Verification items for the finished model (mm, model axes). Give positions to 0.01 mm unless a question says otherwise; leave off trailing zeros. Write each loop counter-clockwise with the first axis right and the second up, starting at its lowest first coordinate (ties: lowest second). Pieces come first, ordered by that corner, then holes. Notation, with made-up numbers: M 12,59 L 21,59 A13 cw 21,83 Z; hole C -31,-34.75 d10. An arc over 180 degrees is marked long. Write item = value, one per line.
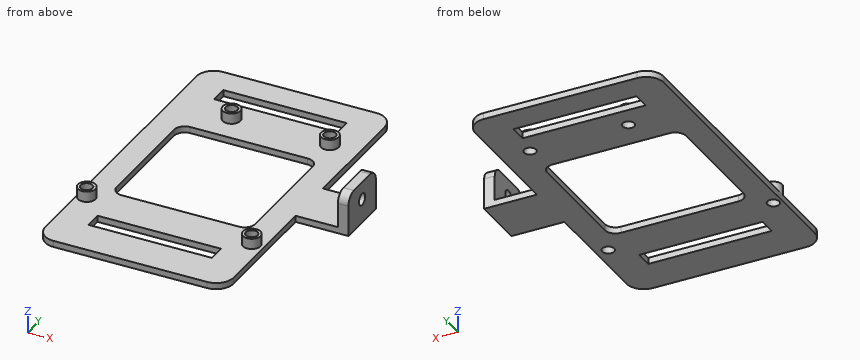
from build123d import *

# Parameters (mm, degrees)
SKETCH_W        = 53.5
SKETCH_H        = 92.8
PAD_DEPTH       = 1.8
SKETCH001_R     = 2.5
PAD001_DEPTH    = 3
SKETCH002_R     = 1.7
POCKET_DEPTH    = 5
SKETCH003_W     = 15
SKETCH003_H     = 1.8
PAD002_DEPTH    = 15
SKETCH004_W     = 39.320262
SKETCH004_H     = 37.514924
POCKET001_DEPTH = 5
FILLET_R        = 5
FILLET001_R     = 5
SKETCH005_W     = 35
SKETCH005_H     = 5
POCKET002_DEPTH = 5
SKETCH006_W     = 3
SKETCH006_H     = 15
PAD003_DEPTH    = 10
SKETCH007_R     = 1.7
POCKET003_DEPTH = 5
FILLET002_R     = 5
FILLET003_R     = 5
FILLET004_R     = 3
FILLET005_R     = 3
FILLET006_R     = 3
FILLET007_R     = 3
FILLET008_R     = 3
FILLET009_R     = 3


with BuildPart() as part:
    # Sketch → Pad (new body)
    with BuildSketch(Plane.XY):
        with Locations((0.1, 0)):
            Rectangle(SKETCH_W, SKETCH_H)
    extrude(amount=PAD_DEPTH)

    # Sketch001 (on Face6 of Pad) → Pad001 (join)
    with BuildSketch(Plane.XY.offset(1.8)):
        with Locations((-9.25, 27.14)):
            Circle(SKETCH001_R)
        with Locations((18.65, 27.14)):
            Circle(SKETCH001_R)
        with Locations((-24.132207, -23.46)):
            Circle(SKETCH001_R)
        with Locations((23.35, -24.76)):
            Circle(SKETCH001_R)
    extrude(amount=PAD001_DEPTH)

    # Sketch002 (on Face12 of Pad001) → Pocket (cut)
    with BuildSketch(Plane.XY.offset(4.8)):
        with Locations((-24.174742, -23.495716)):
            Circle(SKETCH002_R)
        with Locations((-9.25, 27.14)):
            Circle(SKETCH002_R)
        with Locations((18.65, 27.14)):
            Circle(SKETCH002_R)
        with Locations((23.35, -24.764911)):
            Circle(SKETCH002_R)
    extrude(amount=-POCKET_DEPTH, mode=Mode.SUBTRACT)

    # Sketch003 (on Face3 of Pocket) → Pad002 (join)
    with BuildSketch(Plane.YZ.offset(26.85)):
        with Locations((0, 0.9)):
            Rectangle(SKETCH003_W, SKETCH003_H)
    extrude(amount=PAD002_DEPTH)

    # Sketch004 (on Face5 of Pad002) → Pocket001 (cut)
    with BuildSketch(Plane.XY.offset(1.8)):
        Rectangle(SKETCH004_W, SKETCH004_H)
    extrude(amount=-POCKET001_DEPTH, mode=Mode.SUBTRACT)

    # Fillet
    fillet_edges = [part.edges().sort_by_distance(p)[0] for p in [
        (-26.65, 46.4, 0.9),
    ]]
    fillet(fillet_edges, radius=FILLET_R)

    # Fillet001
    fillet001_edges = [part.edges().sort_by_distance(p)[0] for p in [
        (26.85, -46.4, 0.9),
    ]]
    fillet(fillet001_edges, radius=FILLET001_R)

    # Sketch005 → Pocket002 (cut)
    with BuildSketch(Plane.XY.offset(1.8)):
        with Locations((0, -32.91241)):
            Rectangle(SKETCH005_W, SKETCH005_H)
        with Locations((0, 36.086824)):
            Rectangle(SKETCH005_W, SKETCH005_H)
    extrude(amount=-POCKET002_DEPTH, mode=Mode.SUBTRACT)

    # Sketch006 (on Face18 of Pocket001) → Pad003 (join)
    with BuildSketch(Plane.XY.offset(1.8)):
        with Locations((40.35, 0)):
            Rectangle(SKETCH006_W, SKETCH006_H)
    extrude(amount=PAD003_DEPTH)

    # Sketch007 (on Face42 of Pad003) → Pocket003 (cut)
    with BuildSketch(Plane(origin=(38.85, 0, 0), x_dir=(0, -1, 0), z_dir=(-1, 0, 0))):
        with Locations((0, 6.8)):
            Circle(SKETCH007_R)
    extrude(amount=-POCKET003_DEPTH, mode=Mode.SUBTRACT)

    # Fillet002
    fillet002_edges = [part.edges().sort_by_distance(p)[0] for p in [
        (-26.65, -46.4, 0.9),
    ]]
    fillet(fillet002_edges, radius=FILLET002_R)

    # Fillet003
    fillet003_edges = [part.edges().sort_by_distance(p)[0] for p in [
        (26.85, 46.4, 0.9),
    ]]
    fillet(fillet003_edges, radius=FILLET003_R)

    # Fillet004
    fillet004_edges = [part.edges().sort_by_distance(p)[0] for p in [
        (40.35, -7.5, 11.8),
    ]]
    fillet(fillet004_edges, radius=FILLET004_R)

    # Fillet005
    fillet005_edges = [part.edges().sort_by_distance(p)[0] for p in [
        (40.35, 7.5, 11.8),
    ]]
    fillet(fillet005_edges, radius=FILLET005_R)

    # Fillet006
    fillet006_edges = [part.edges().sort_by_distance(p)[0] for p in [
        (19.660131, 18.757462, 0.9),
    ]]
    fillet(fillet006_edges, radius=FILLET006_R)

    # Fillet007
    fillet007_edges = [part.edges().sort_by_distance(p)[0] for p in [
        (-19.660131, 18.757462, 0.9),
    ]]
    fillet(fillet007_edges, radius=FILLET007_R)

    # Fillet008
    fillet008_edges = [part.edges().sort_by_distance(p)[0] for p in [
        (19.660131, -18.757462, 0.9),
    ]]
    fillet(fillet008_edges, radius=FILLET008_R)

    # Fillet009
    fillet009_edges = [part.edges().sort_by_distance(p)[0] for p in [
        (-19.660131, -18.757462, 0.9),
    ]]
    fillet(fillet009_edges, radius=FILLET009_R)


solid = part.part
1) Material ranges on probe 1 along Y at (x, z) = (-9.25, 1.6); probe 2 along X at (y, z) = (27, 4.5); probe 3 along X at (y, z) = (-15, 1.25), recorded low to high. Write a range as from..to.
From the geometry:
probe_1 = -46.4..-35.41, -30.41..-18.76, 18.76..25.44, 28.84..33.59, 38.59..46.4
probe_2 = -11.75..-10.94, -7.56..-6.75, 16.15..16.96, 20.34..21.15
probe_3 = -26.65..-19.66, 19.66..26.85
2) Cross-section at D-D on y = -28.5. Record the boundary of the cut face in (x, z).
From the geometry:
outline = M -26.65,0 L 26.85,0 L 26.85,1.8 L -26.65,1.8 Z
3) Depth check by flat-ended pin: P1, Ø1.5, axis at x = 24, y = -25.5, coming from the +Z side; P2, Ø5, axis at x = -13, z = 6, coming from the +Y side. Enter the tip coordinate at first touch or a pass-through.
From the geometry:
P1 = 4.8
P2 = 29.1
4) Cross-section at B-B on y = 0. Record the boundary of the cut face in (x, z).
From the geometry:
outline = M -26.65,0 L -19.66,0 L -19.66,1.8 L -26.65,1.8 Z; M 19.66,0 L 41.85,0 L 41.85,5.1 L 38.85,5.1 L 38.85,1.8 L 19.66,1.8 Z; M 38.85,8.5 L 41.85,8.5 L 41.85,11.8 L 38.85,11.8 Z
5) Cross-section at C-C on x = 24. Record the boundary of the cut face in (y, z), plus the area to 3 significant figures.
From the geometry:
outline = M -45.91,0 L -26.34,0 L -26.34,4.8 L -27.17,4.8 L -27.17,1.8 L -45.91,1.8 Z; M -23.19,0 L 45.91,0 L 45.91,1.8 L -22.35,1.8 L -22.35,4.8 L -23.19,4.8 Z
area = 165 mm^2
6) Cross-section at A-A on x = -9.25. Record the boundary of the cut face in (y, z).
From the geometry:
outline = M -46.4,0 L -35.41,0 L -35.41,1.8 L -46.4,1.8 Z; M -30.41,0 L -18.76,0 L -18.76,1.8 L -30.41,1.8 Z; M 18.76,0 L 25.44,0 L 25.44,4.8 L 24.64,4.8 L 24.64,1.8 L 18.76,1.8 Z; M 28.84,0 L 33.59,0 L 33.59,1.8 L 29.64,1.8 L 29.64,4.8 L 28.84,4.8 Z; M 38.59,0 L 46.4,0 L 46.4,1.8 L 38.59,1.8 Z
